Can you work these out from the drawing? Everything is in mm from the part's minimum corner. A direction names the side the tool comes from. Round coordinates to 2 decimals unless told otherwise and drop trailing zeros. Write each loop counter-clockwise with the first axis right and the second up, starting at its lowest first coordinate (ties: lowest second). Pieces come first, ordered by that corner, then holes. Notation, with made-up numbers: (14, 7) -> (30, 7) arc R26 ccw to (30, 39) -> close; hole circle Ø8 at (52.5, 88.5). An arc over 180 degrees is marked (long way). Answer as CSV lines item,"result". Start each with the question number.
Q1. If we mould it in two halves opening along X, with no side actions, what happens to the marked faces 1, 2 and 3? For each: pulls with the +X half, pulls with the -X half, needs draft (parallel to the pull), parting line crosses it, or undercut.
Q2. Will these pins go through, and if not, where does the flat tip stop? pin 1 Ø2.5 at (x, y) = (9, 64) entering from -Z; pin 2 Ø12 at (y, z) = (84.5, 33) entering from -X.
Q3. Imagine slicing it at D-D on y = 61. Please give me the cut outline in (x, z).
Q4. Imagine slicing it at C-C on x = 1.5. Please give me the cut outline in (y, z).
Q5. Imagine slicing it at B-B on y = 49.53. Please give me the cut outline in (x, z) (1 decimal), and give its area (3 significant figures).
Q6. Imagine slicing it at A-A on z = 23. Please give me the cut outline in (x, y), and give its area (3 significant figures).
Q7. For the marked faces 4 and 5, which set-ups out of +Z, -Z, +X, -X, +Y, -Y let a thin tool reach every point of the face, with its end or its side?
Q8. If I drill on line 1 (X direction, y = 92, z = 48); line 2 (Z direction, x = 0.9, y = 49.53) (1 decimal); line 3 (Y direction, x = 2.5, z = 46), over which ranges is the centre line in solid material (lowest first)? Write a range as [from, to].
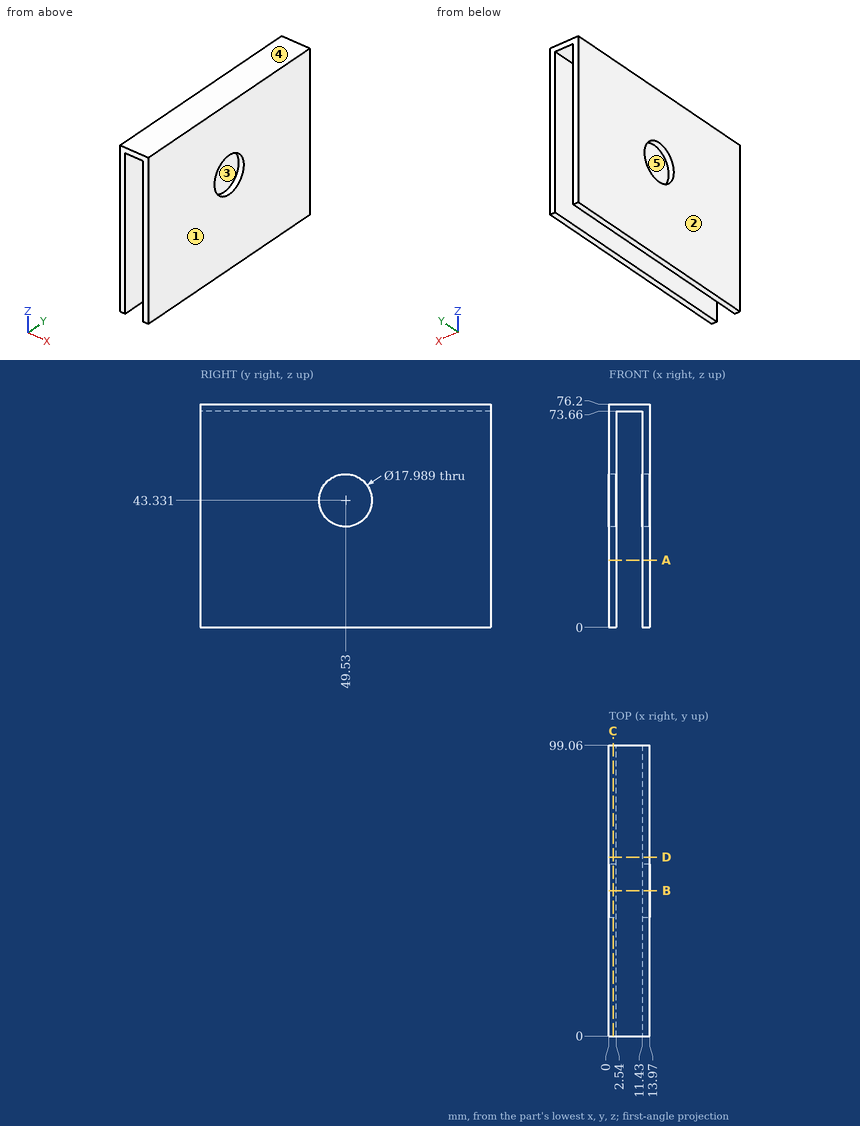
Checks:
1,face 1,"pulls with the +X half"
1,face 2,"pulls with the -X half"
1,face 3,"undercut"
2,pin 1,"z = 73.66"
2,pin 2,"x = 0"
3,outline,"(0, 0) -> (2.54, 0) -> (2.54, 73.66) -> (11.43, 73.66) -> (11.43, 0) -> (13.97, 0) -> (13.97, 76.2) -> (0, 76.2) -> close"
4,outline,"(0, 0) -> (99.06, 0) -> (99.06, 76.2) -> (0, 76.2) -> close; hole circle Ø17.99 at (49.53, 43.33)"
5,outline,"(0, 0) -> (2.5, 0) -> (2.5, 34.3) -> (0, 34.3) -> close; (0, 52.3) -> (2.5, 52.3) -> (2.5, 73.7) -> (11.4, 73.7) -> (11.4, 52.3) -> (14, 52.3) -> (14, 76.2) -> (0, 76.2) -> close; (11.4, 0) -> (14, 0) -> (14, 34.3) -> (11.4, 34.3) -> close"
5,area,"318 mm^2"
6,outline,"(0, 0) -> (2.54, 0) -> (2.54, 99.06) -> (0, 99.06) -> close; (11.43, 0) -> (13.97, 0) -> (13.97, 99.06) -> (11.43, 99.06) -> close"
6,area,"503 mm^2"
7,face 4,"+Z, +X, -X, +Y, -Y"
7,face 5,"-Z, +Y, -Y"
8,line 1,"[0, 2.54], [11.43, 13.97]"
8,line 2,"[0, 34.3], [52.3, 76.2]"
8,line 3,"[0, 40.94], [58.12, 99.06]"
